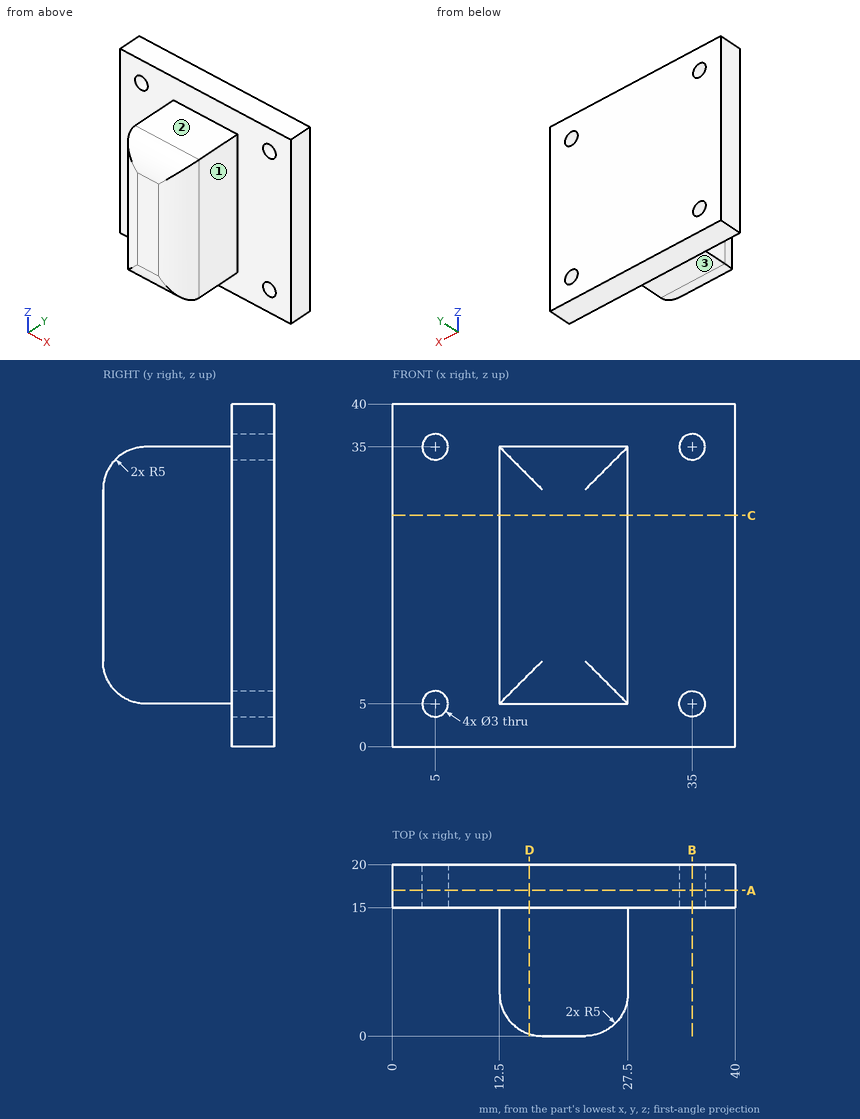
The drawing under review shows one solid part. Ordinate dimensions are in mm from its lowest x, y, z. A direction names the side the tool comes from. Give positions to 0.01 mm unless a question says otherwise; leave off trailing zeros. Write each loop counter-clockwise with the first axis right and the second up, starting at its lowest first coordinate (ties: lowest second). Pieces come first, ordered by that corner, then holes. Notation, with made-up numbers: M -11.75,63 L 0.25,63 A23 cw 0.25,78 Z; hole C 72,25.25 d9. An arc over 180 degrees is marked long. Write each question's results on one line, items separated by ' | '. Start each with the question number.
1. For probe 1 along Z at (x, y) = (5, 18.3); probe 2 along X at (y, z) = (11.75, 34); probe 3 along Y at (x, z) = (34, 37), list the stretches that pass through material, from the lowest coordinate up. Write a range as [from, to].
2. For the marked faces 1, 2 and 3, list the 3-axis set-ups (+Z, -Z, +X, -X, +Y, -Y) from which the entire face can be reached by the end or side of a thin tool; tool diameter is ignored.
3. We need section B-B (x = 35). Write out the cut boundary in (y, z).
4. We need section C-C (z = 27). Write out the cut boundary in (x, y), and give its area (3 significant figures).
5. We need section D-D (x = 16). Write out the cut boundary in (y, z).
6. We need section A-A (y = 17). Write out the cut boundary in (x, z), and give its area (3 significant figures).
7. Insertion check: pin 1 Ø5 at (x, z) = (5, 5) entering from -Y; pin 2 Ø2.5 at (x, z) = (35, 35) entering from +Y (3 decimals); pin 3 Ø8 at (y, z) = (9.5, 21.5) entering from -X; pin 4 Ø8 at (y, z) = (9.5, 15) entering from +X. Each pin has a flat end and moves straight along its axis. Give the tip position at first contact, or say it passes through.
Results found:
1) probe 1: z = [0, 3.5], [6.5, 33.5], [36.5, 40] | probe 2: x = [12.5, 27.5] | probe 3: y = [15, 20]
2) face 1: +Z, -Z, +X, -Y | face 2: +Z, +X, -X, -Y | face 3: -Z, +X, -X, -Y
3) outline: M 15,0 L 20,0 L 20,3.5 L 15,3.5 Z; M 15,6.5 L 20,6.5 L 20,33.5 L 15,33.5 Z; M 15,36.5 L 20,36.5 L 20,40 L 15,40 Z
4) outline: M 0,15 L 12.5,15 L 12.5,5 A5 ccw 17.5,0 L 22.5,0 A5 ccw 27.5,5 L 27.5,15 L 40,15 L 40,20 L 0,20 Z | area: 414 mm^2
5) outline: M 0.23,8.5 A5 ccw 5,5 L 15,5 L 15,0 L 20,0 L 20,40 L 15,40 L 15,35 L 5,35 A5 ccw 0.23,31.5 Z
6) outline: M 0,0 L 40,0 L 40,40 L 0,40 Z; hole C 5,5 d3; hole C 5,35 d3; hole C 35,5 d3; hole C 35,35 d3 | area: 1,570 mm^2
7) pin 1: stops at y = 15 | pin 2: passes through | pin 3: stops at x = 12.5 | pin 4: stops at x = 27.5
